Source: three-view drawing plus pictorial views. Frame: mm from the lowest corner of the part. A direction names the side the tool comes from. Round coordinates to 2 decimals unless told otherwise and drop trailing zeros. Loops run counter-clockwise (first coordinate to the right, second up) from the corner with the lowest first, then second, coordinate; pieces in that order, holes last. Notation, with made-up numbers: M 87.5,12.5 L 130.5,12.5 A21 ccw 130.5,21.5 Z; hole C 89.25,20 d6. An arc over 180 degrees is marked long. Answer as a JSON object with one key per item and string values.
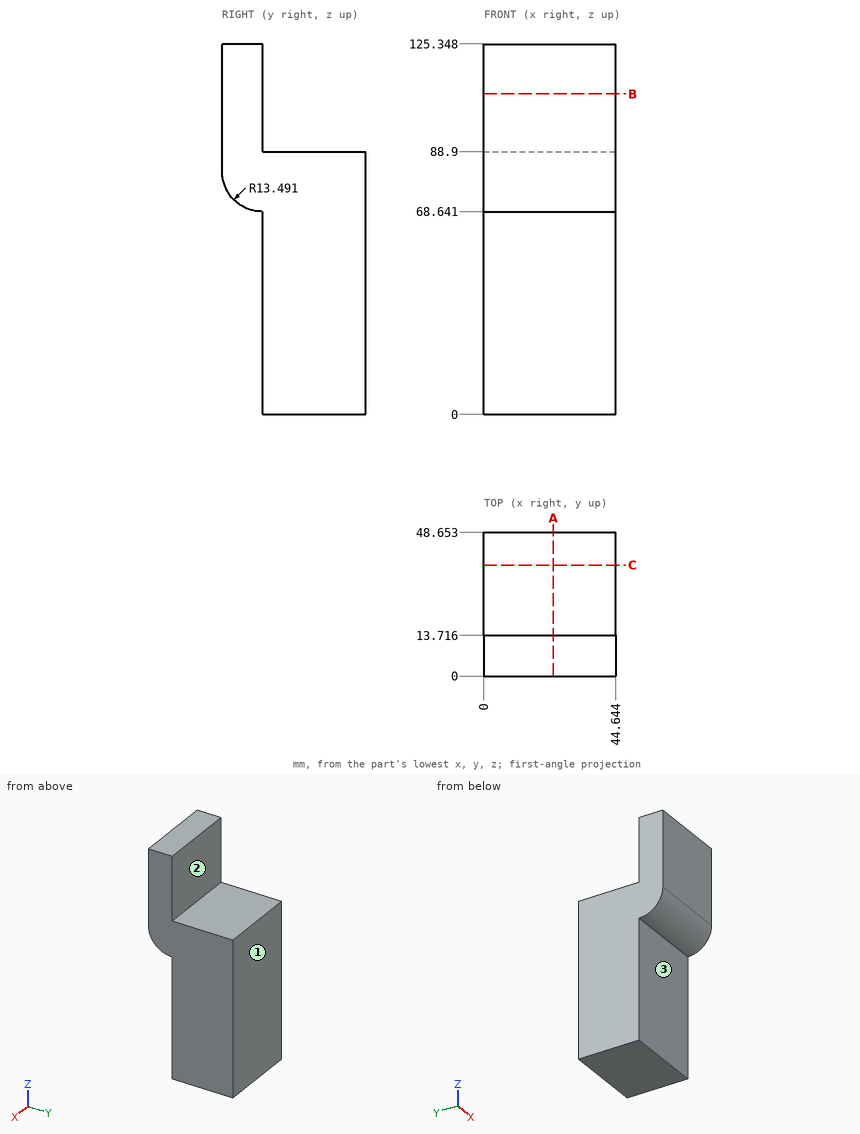
1) Set-up query: the marked faces 1, 2 and 3. Return all of +Z, -Z, +X, -X, +Y, -Y with unobstructed straight access to the full face (end or side cutting, diameter ignored); none if empty.
Geometry results:
{"face 1": "+Z, -Z, +X, -X, +Y", "face 2": "+Z, +X, -X, +Y", "face 3": "-Z, +X, -X, -Y"}
2) Line query: probe 1 along Y at (x, z) = (7, 22.5); probe 2 along Z at (x, y) = (32.5, 13.5); probe 3 along Z at (x, y) = (33.5, 15.5). Output: solid intervals per line, ascending.
Geometry results:
{"probe 1": "13.72 to 48.65", "probe 2": "68.64 to 125.35", "probe 3": "0 to 88.9"}
3) First-contact query: pin 1 (18 mm diameter, centred on x = 26.5, z = 108.5, fed in from +Y); pin 2 (10.5 mm diameter, centred on x = 24, y = 25, fed in from +Z); pin 3 (4 mm diameter, centred on x = 25.5, z = 54, fed in from -Y); pin 4 (3 mm diameter, centred on y = 11, z = 49, fed in from -X). Flat tips, straight axial feed; report the tip coordinate or a pass-through.
Geometry results:
{"pin 1": "y = 13.72", "pin 2": "z = 88.9", "pin 3": "y = 13.72", "pin 4": "through"}
4) Cut plane A-A on x = 23.5. Return the cut outline in (y, z), and give its area (3 significant figures).
Geometry results:
{"outline": "M 0,82.13 A13.49 ccw 13.49,68.64 L 13.72,68.64 L 13.72,0 L 48.65,0 L 48.65,88.9 L 13.72,88.9 L 13.72,125.35 L 0,125.35 Z", "area": "3,840 mm2"}
5) Cut plane C-C on y = 37.5. Return the cut outline in (x, z), and give its area (3 significant figures).
Geometry results:
{"outline": "M 0,0 L 44.64,0 L 44.64,88.9 L 0,88.9 Z", "area": "3,970 mm2"}
6) Cut plane B-B on z = 108.5. Return the cut outline in (x, y).
Geometry results:
{"outline": "M 0,0 L 44.64,0 L 44.64,13.72 L 0,13.72 Z"}
